Design review of the part shown in the three views and the two pictorial views. Dimensions are in mm from the part's minimum x, y and z. A direction names the side the tool comes from. Give positions to 0.01 mm unless a question says otherwise; leave off trailing zeros. Loops run counter-clockwise (first coordinate to the right, second up) from the corner with the lowest first, then second, coordinate; pieces in that order, holes last. Notation, with made-up numbers: (75, 53) -> (106, 53) arc R27 ccw to (106, 88) -> close; hole circle Ø2 at (73, 61). An arc over 180 degrees is marked (long way). Use CSV: the item, a comma, the result in double quotes. Start each with the question number.
Item 1: For the marked faces 4, 5, 6, 7 and 8, list the 3-axis set-ups (+Z, -Z, +X, -X, +Y, -Y) from which the entire face can be reached by the end or side of a thin tool; tool diameter is ignored.
Item 2: We need section A-A (z = 10). State the section outline as (x, y) points.
Item 3: Wall thickness on line 1 along Z through (x, y) = (3, 0.75); line 2 along X through (y, z) = (0.85, 59); line 3 along Y through (x, z) = (25, 29): over which ranges is each line inside the solid? List them lowest first. Write a range as from..to.
Item 4: The part is to be moulded in two halves that separate along Z. For the marked faces 1, 2 and 3, say which applies: +Z half, -Z half, draft (parallel to the pull), parting line (faces both ways), or undercut.
Item 5: We need section D-D (x = 3). State the section outline as (y, z) points, plus the area to 3 significant figures.
Item 6: We need section C-C (x = 19). State the section outline as (y, z) points, plus the area to 3 significant figures.
Item 7: Clearance check with flat-ended pins moving along their axes: pin 1 (3 mm diameter, centred on x = 19, y = 8, fed in from +Z); pin 2 (3.5 mm diameter, centred on y = 5.5, z = 11.5, fed in from -X); pin 3 (6 mm diameter, centred on x = 48, y = 6.5, fed in from -Z). State where each tip first meets the part, or that it passes through.
Item 8: We need section B-B (y = 8). State the section outline as (x, z) points.
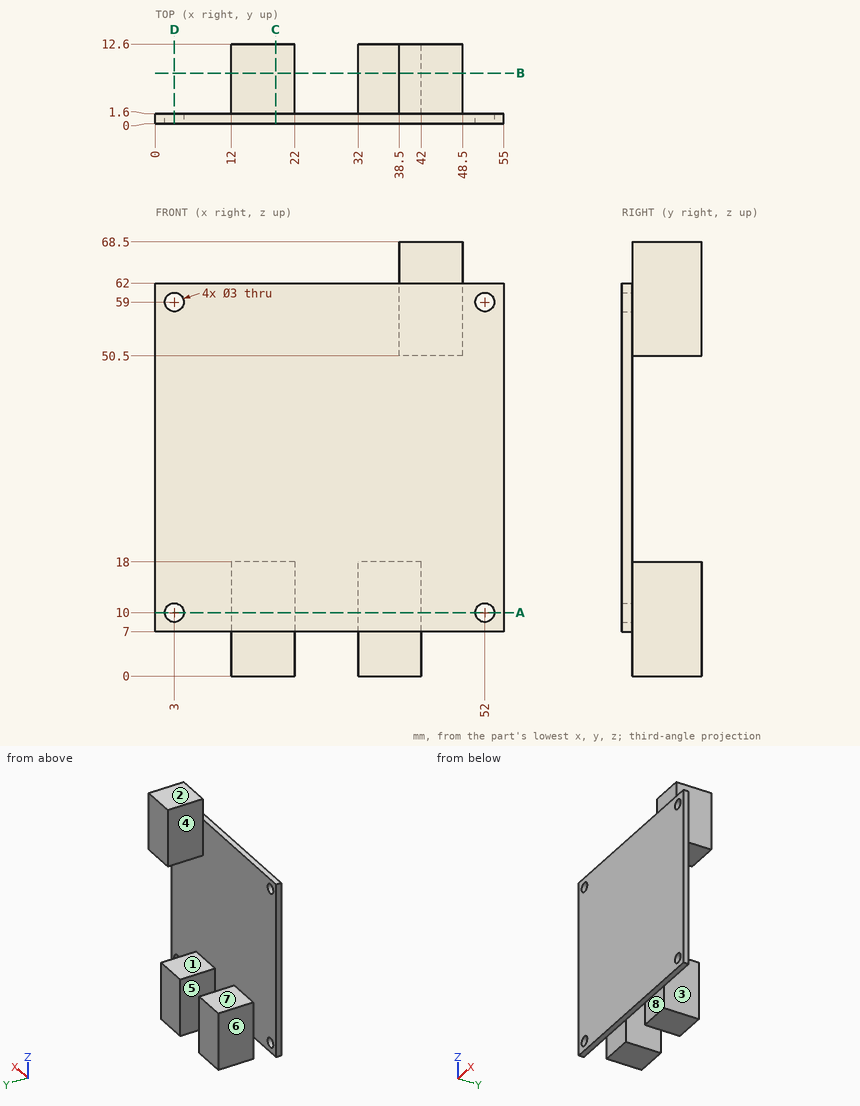
Results found:
1,face 4,"+Z, -X, +Y"
1,face 5,"+Z, -Z, +Y"
1,face 6,"+Z, -Z, -X, +Y"
1,face 7,"+Z, +X, -X, +Y"
1,face 8,"-Z, +X, -X, -Y"
2,outline,"(0, 0) -> (1.5, 0) -> (1.5, 1.6) -> (0, 1.6) -> close; (4.5, 0) -> (50.5, 0) -> (50.5, 1.6) -> (42, 1.6) -> (42, 12.6) -> (32, 12.6) -> (32, 1.6) -> (22, 1.6) -> (22, 12.6) -> (12, 12.6) -> (12, 1.6) -> (4.5, 1.6) -> close; (53.5, 0) -> (55, 0) -> (55, 1.6) -> (53.5, 1.6) -> close"
3,line 1,"7..8.5, 11.5..57.5, 60.5..62"
3,line 2,"0..1.5, 4.5..50.5, 53.5..55"
3,line 3,"0..1.6"
4,face 1,"undercut"
4,face 2,"+Z half"
4,face 3,"draft"
5,outline,"(0, 7) -> (1.6, 7) -> (1.6, 8.5) -> (0, 8.5) -> close; (0, 11.5) -> (1.6, 11.5) -> (1.6, 57.5) -> (0, 57.5) -> close; (0, 60.5) -> (1.6, 60.5) -> (1.6, 62) -> (0, 62) -> close"
5,area,"78.4 mm²"
6,outline,"(0, 7) -> (1.6, 7) -> (1.6, 0) -> (12.6, 0) -> (12.6, 18) -> (1.6, 18) -> (1.6, 62) -> (0, 62) -> close"
6,area,"286 mm²"
7,pin 1,"z = 18"
7,pin 2,"x = 12"
7,pin 3,"z = 50.5"
8,outline,"(12, 0) -> (22, 0) -> (22, 18) -> (12, 18) -> close; (32, 0) -> (42, 0) -> (42, 18) -> (32, 18) -> close; (38.5, 50.5) -> (48.5, 50.5) -> (48.5, 68.5) -> (38.5, 68.5) -> close"
